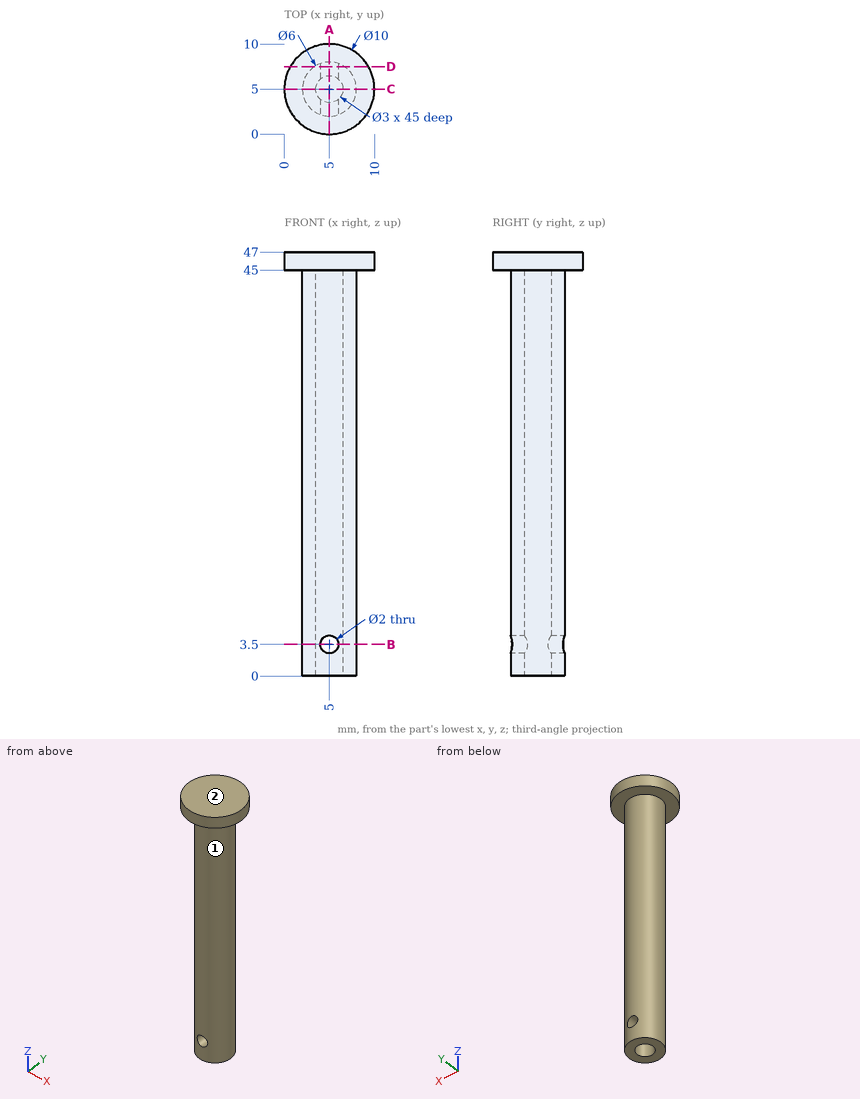
Print and shaded views of the part. All mm, measured from the part's lowest x, y and z. A direction names the side the tool comes from. Round coordinates to 2 decimals unless told otherwise and drop trailing zeros. Write each loop counter-clockwise with the first axis right and the second up, starting at its lowest first coordinate (ties: lowest second). Pieces come first, ordered by that corner, then holes. Notation, with made-up numbers: (65, 29) -> (103, 29) arc R19 cw to (103, 39) -> close; hole circle Ø1 at (41.25, 74). An arc over 180 degrees is marked (long way). Answer in a Markdown table with one row per item. Add a question column.
Item 1: Saw through at D-D, the plane y = 7.5. Write the cut outline in (x, z).
Item 2: Drop flat-ended pins along their axis: pin 1 Ø4 at (x, z) = (5, 11.5) entering from -Y; pin 2 Ø2.5 at (x, z) = (5, 3.5) entering from +Y; pin 3 Ø2 at (y, z) = (5, 28.5) entering from +X. Give the stop position or say it passes through.
Item 3: Which spindle directions (+Z, -Z, +X, -X, +Y, -Y) get a long thin tool onto all of the face, cutting with end or side? Do the marked faces 1 and 2. Say none if no direction does.
Item 4: Saw through at A-A, the plane x = 5. Write the cut outline in (y, z).
Item 5: Saw through at B-B, the plane z = 3.5. Write the cut outline in (x, y), then the cut area to 3 significant figures.
Item 6: Saw through at C-C, the plane y = 5. Write the cut outline in (x, z).
Item 7: Drill centre lines: line 1 (Z direction, x = 5, y = 2.95); line 2 (Z direction, x = 9, y = 3.75); line 3 (X direction, y = 2.4, z = 3.5). Where is each one in solid material? Low to high. Write a range as from..to.
Findings below:
| question | item | result |
|---|---|---|
| 1 | outline | (0.67, 45) -> (3.34, 45) -> (3.34, 0) -> (6.66, 0) -> (6.66, 45) -> (9.33, 45) -> (9.33, 47) -> (0.67, 47) -> close; hole circle Ø2 at (5, 3.5) |
| 2 | pin 1 | stops at y = 2 |
| 2 | pin 2 | stops at y = 8 |
| 2 | pin 3 | stops at x = 8 |
| 3 | face 1 | -Z |
| 3 | face 2 | +Z, +X, -X, +Y, -Y |
| 4 | outline | (0, 45) -> (2, 45) -> (2, 4.5) -> (3.5, 4.5) -> (3.5, 45) -> (6.5, 45) -> (6.5, 4.5) -> (8, 4.5) -> (8, 45) -> (10, 45) -> (10, 47) -> (0, 47) -> close; (2, 0) -> (3.5, 0) -> (3.5, 2.5) -> (2, 2.5) -> close; (6.5, 0) -> (8, 0) -> (8, 2.5) -> (6.5, 2.5) -> close |
| 5 | outline | (4, 2.17) -> (4, 3.88) arc R1.5 cw to (4, 6.12) -> (4, 7.83) arc R3 ccw to start; (6, 2.17) arc R3 ccw to (6, 7.83) -> (6, 6.12) arc R1.5 cw to (6, 3.88) -> close |
| 5 | area | 15.0 mm^2 |
| 6 | outline | (0, 45) -> (2, 45) -> (2, 0) -> (3.5, 0) -> (3.5, 45) -> (6.5, 45) -> (6.5, 0) -> (8, 0) -> (8, 45) -> (10, 45) -> (10, 47) -> (0, 47) -> close |
| 7 | line 1 | z = 0..2.5, 4.5..47 |
| 7 | line 2 | z = 45..47 |
| 7 | line 3 | x = 3.5..4, 6..6.5 |
